Can you work these out from the model? Positions are in its coordinate system, mm. Face numbers are marked on the shaded views. A direction names the side the tool comes from. Give positions to 0.01 mm unless a question says otherwise; leave off trailing zeros. Loops run counter-clockwise (first coordinate to the right, second up) from the corner with the lowest first, then second, coordinate; pieces in that order, holes last. Notation, with made-up numbers: M -26.5,50.25 L 32.5,50.25 A21 cw 32.5,58.25 Z; hole C 17.25,46 d10. An arc over 180 degrees is marked long. Use CSV: the item, a comma, the result in double quotes.
Autodesk Inventor part; units mm, degrees
ref_plane "YZ Plane" through (0, 0, 0) normal (1, 0, 0) x (0, 1, 0)
ref_plane "XZ Plane" through (0, 0, 0) normal (0, 1, 0) x (-1, 0, 0)
ref_plane "XY Plane" through (0, 0, 0) normal (0, 0, 1) x (1, 0, 0)
sketch "Sketch1" plane through (0, 0, 0) normal (0, 1, 0) x (-1, 0, 0)
  line L0 (0, 0) -> (-38.1, 0)
  line L1 (-38.1, 0) -> (-38.1, -82.55)
  line L2 (-38.1, -82.55) -> (0, -82.55)
  line L3 (0, -82.55) -> (0, 0)
  circle A0 centre (-22.6822, 4.7752) radius 3.175
  circle A1 centre (-9.9822, 4.7752) radius 3.175
  line L4 (0, 0) -> (-38.1, 0)
  line L5 (-38.1, 0) -> (-38.1, 12.7)
  line L6 (-38.1, 12.7) -> (0, 12.7)
  line L7 (0, 12.7) -> (0, 0)
  dimension "d0" = 38.1
  dimension "d1" = 82.55
  dimension "d24" = 6.35
  dimension "d25" = 15.4178
  dimension "d27" = 6.35
  dimension "d28" = 12.7
  dimension "d29" = 12.7
  dimension "d30" = 7.9248
extrude "Extrusion1" add sketch "Sketch1" along normal blind 12.7
sketch "Sketch2" plane through (0, 12.7, 0) normal (0, 1, 0) x (1, 0, 0)
  circle A0 centre (19.3548, 58.7375) radius 16.51
  line L0 (0, 82.55) -> (0, 0)
  line L1 (38.1, 82.55) -> (0, 82.55)
  point P0 (9.6774, 7.9375)
  dimension "d8" = 33.02
  dimension "d23" = 9.6774
extrude "Extrusion2" add sketch "Sketch2" along normal blind 50.8 and the other way blind 76.2
sketch "Sketch3" plane through (19.3548, 63.5, -58.7375) normal (0, 1, 0) x (1, 0, 0)
  circle A0 centre (0, 0) radius 13.0175
  point P0 (-19.3548, -58.7375)
  dimension "d17" = 26.035
extrude "Extrusion3" cut sketch "Sketch3" against normal blind 41.91
sketch "Sketch4" plane through (19.3548, 21.59, -58.7375) normal (0, 1, 0) x (1, 0, 0)
  circle A0 centre (0, 0) radius 16
  point P0 (-19.3548, -58.7375)
  dimension "d20" = 31.9999
extrude "Extrusion4" cut sketch "Sketch4" against normal blind 59.69
properties part number "Flip up and down motion motor mount"
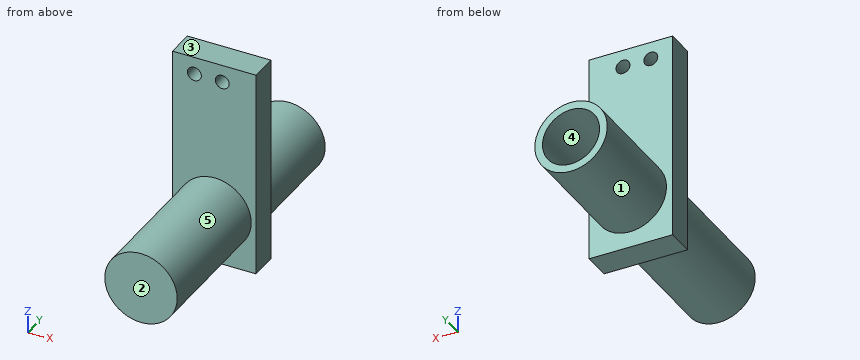
Q1. Please list where these lines run through material, in increasing order: L1, parallel to Y at x = 26, z = -39; L2, parallel to Z at x = 25, y = -19; L3, parallel to Z at x = 27, y = 28. Write a range as from..to.
Model answer:
L1,"0..12.7"
L2,"-74.25..-73.71, -43.77..-43.22"
L3,"-73.37..-69.27, -48.2..-44.1"
Q2. I want a section at C-C, the plane y = 55.5. Please give me the cut outline in (x, z) (1 decimal), then the cut area to 3 significant figures.
Model answer:
outline,"C 19.4,-58.7 d33; hole C 19.4,-58.7 d26"
area,"324 mm2"
Q3. I want a section at D-D, the plane z = -54. Please give me the cut outline in (x, y), then the cut area to 3 significant figures.
Model answer:
outline,"M 0,0 L 3.54,0 L 3.54,-63.5 L 35.17,-63.5 L 35.17,0 L 38.1,0 L 38.1,12.7 L 35.17,12.7 L 35.17,63.5 L 31.48,63.5 L 31.48,21.59 L 34.64,21.59 L 34.64,-38.1 L 4.07,-38.1 L 4.07,21.59 L 7.23,21.59 L 7.23,63.5 L 3.54,63.5 L 3.54,12.7 L 0,12.7 Z"
area,"1,260 mm2"
Q4. If we mould it in two halves opening along Z, with no side actions, what happens to the marked faces 3, 4 and 5? For each: released by +Z, released by -Z, zero draft, split by the parting line, or undercut.
Model answer:
face 3,"released by +Z"
face 4,"undercut"
face 5,"split by the parting line"
Q5. I'm going to push flat-ended pins straight in: P1, Ø1, axis at x = 7.5, y = -43, coming from the -Z side; P2, Ø1, axis at x = 27, z = -50, coming from the +Y side; P3, Ø6, axis at x = 33, z = -70, coming from the +Y side; P4, Ø8.5, axis at x = 9.98, z = 4.78, coming from the +Y side. Where does each tip first touch, or does it pass through?
Model answer:
P1,"z = -70.72"
P2,"y = -38.1"
P3,"y = 63.5"
P4,"y = 12.7"
Q6. I want a section at A-A, the plane x = 22. Please give me the cut outline in (y, z), then the cut area to 3 significant figures.
Model answer:
outline,"M -63.5,-75.03 L 0,-75.03 L 0,-82.55 L 12.7,-82.55 L 12.7,-75.03 L 63.5,-75.03 L 63.5,-71.48 L 21.59,-71.48 L 21.59,-74.52 L -38.1,-74.52 L -38.1,-42.96 L 21.59,-42.96 L 21.59,-45.99 L 63.5,-45.99 L 63.5,-42.44 L 12.7,-42.44 L 12.7,1.67 L 0,1.67 L 0,-42.44 L -63.5,-42.44 Z; M 0,7.88 L 12.7,7.88 L 12.7,12.7 L 0,12.7 Z"
area,"1,900 mm2"
Q7. I want a section at B-B, the plane x = 15.5. Please give me the cut outline in (y, z), then the cut area to 3 significant figures.
Model answer:
outline,"M -63.5,-74.79 L 0,-74.79 L 0,-82.55 L 12.7,-82.55 L 12.7,-74.79 L 63.5,-74.79 L 63.5,-71.17 L 21.59,-71.17 L 21.59,-74.27 L -38.1,-74.27 L -38.1,-43.21 L 21.59,-43.21 L 21.59,-46.3 L 63.5,-46.3 L 63.5,-42.68 L 12.7,-42.68 L 12.7,12.7 L 0,12.7 L 0,-42.68 L -63.5,-42.68 Z"
area,"1,980 mm2"
Q8. For the marked faces 1 and 2, which set-ups out of +Z, -Z, +X, -X, +Y, -Y let a thin tool reach every point of the face, with its end or its side?
Model answer:
face 1,"+Y"
face 2,"+Z, -Z, +X, -X, -Y"
